Input: part model. Units: mm. Frame: model coordinates. A direction names the side the tool comes from. Coordinates: 2 decimals unless noted, no trailing zeros. Write each loop counter-clockwise with the first axis right and the second up, starting at its lowest first coordinate (ties: lowest second). Pieces come first, ordered by that corner, then holes.
1) Section query A-A (y = 12.5). Output: boundary loops of the cut face in (x, z).
2) Set-up query: faces 1 (the cylindrical face through (-1.08, -10.39, -4.88)), 2 (the cylindrical face through (-0.59, 12.89, 4.46)). Return all of +Z, -Z, +X, -X, +Y, -Y with unobstructed straight access to the full face (end or side cutting, diameter ignored); none if empty.
3) Section query B-B (y = -10.5). Output: boundary loops of the cut face in (x, z), then the cut area to 3 significant figures.
4) Line query: L1, parallel to Z at x = 0, y = -5; L2, parallel to Z at x = 0, y = 3.5; L3, parallel to X at y = -10, z = -0.75. Output: solid intervals per line, ascending.
5) Pin query (flat end, axial travel): pin 1 Ø5 at (x, y) = (-0.5, -12.5) entering from +Z; pin 2 Ø5 at (y, z) = (8.5, 2) entering from -X; pin 3 Ø3 at (x, z) = (-1.5, 4) entering from -Y; pin 4 Ø4 at (x, z) = (-1.5, 5.5) entering from +Y. Return the tip coordinate at first contact, or that it passes through.
from build123d import *

# Parameters (mm, degrees)
F0_R        = 7
F0_R_2      = 6.5
F0_R_3      = 6
F0_R_4      = 5.5
F0_R_5      = 5
F0_R_6      = 4.5
F0_R_7      = 4
F1_DEPTH    = 2
F2_DEPTH    = 4.5
F3_DEPTH    = 7
F4_DEPTH    = 9.5
F5_DEPTH    = 12
F6_DEPTH    = 14.5
F7_DEPTH    = 17
F8_R        = 3.25
F9_DEPTH    = 17
F10_SIZE2   = 0.692820323
F10_SIZE    = 0.4
F10_2_SIZE2 = 0.692820323
F10_2_SIZE  = 0.4
F10_3_SIZE2 = 0.692820323
F10_3_SIZE  = 0.4
F10_4_SIZE2 = 0.692820323
F10_4_SIZE  = 0.4
F10_5_SIZE2 = 0.692820323
F10_5_SIZE  = 0.4
F10_6_SIZE2 = 0.692820323
F10_6_SIZE  = 0.4


with BuildPart() as f1:
    # F0 (on Front) → F1 (new body)
    with BuildSketch(Plane.XZ):
        Circle(F0_R)
        Circle(F0_R_2, mode=Mode.SUBTRACT)
        Circle(F0_R_2)
        Circle(F0_R_3, mode=Mode.SUBTRACT)
        Circle(F0_R_3)
        Circle(F0_R_4, mode=Mode.SUBTRACT)
        Circle(F0_R_4)
        Circle(F0_R_5, mode=Mode.SUBTRACT)
        Circle(F0_R_5)
        Circle(F0_R_6, mode=Mode.SUBTRACT)
        Circle(F0_R_6)
        Circle(F0_R_7, mode=Mode.SUBTRACT)
        Circle(F0_R_7)
    extrude(amount=F1_DEPTH)

    # F0 (on Front) → F2 (join, through all)
    with BuildSketch(Plane.XZ):
        Circle(F0_R_2)
        Circle(F0_R_3, mode=Mode.SUBTRACT)
        Circle(F0_R_3)
        Circle(F0_R_4, mode=Mode.SUBTRACT)
        Circle(F0_R_4)
        Circle(F0_R_5, mode=Mode.SUBTRACT)
        Circle(F0_R_5)
        Circle(F0_R_6, mode=Mode.SUBTRACT)
        Circle(F0_R_6)
        Circle(F0_R_7, mode=Mode.SUBTRACT)
        Circle(F0_R_7)
    extrude(amount=F2_DEPTH)

    # F0 (on Front) → F3 (join, through all)
    with BuildSketch(Plane.XZ):
        Circle(F0_R_3)
        Circle(F0_R_4, mode=Mode.SUBTRACT)
        Circle(F0_R_4)
        Circle(F0_R_5, mode=Mode.SUBTRACT)
        Circle(F0_R_5)
        Circle(F0_R_6, mode=Mode.SUBTRACT)
        Circle(F0_R_6)
        Circle(F0_R_7, mode=Mode.SUBTRACT)
        Circle(F0_R_7)
    extrude(amount=F3_DEPTH)

    # F0 (on Front) → F4 (join, through all)
    with BuildSketch(Plane.XZ):
        Circle(F0_R_4)
        Circle(F0_R_5, mode=Mode.SUBTRACT)
        Circle(F0_R_5)
        Circle(F0_R_6, mode=Mode.SUBTRACT)
        Circle(F0_R_6)
        Circle(F0_R_7, mode=Mode.SUBTRACT)
        Circle(F0_R_7)
    extrude(amount=F4_DEPTH)

    # F0 (on Front) → F5 (join, through all)
    with BuildSketch(Plane.XZ):
        Circle(F0_R_5)
        Circle(F0_R_6, mode=Mode.SUBTRACT)
        Circle(F0_R_6)
        Circle(F0_R_7, mode=Mode.SUBTRACT)
        Circle(F0_R_7)
    extrude(amount=F5_DEPTH)

    # F0 (on Front) → F6 (join, through all)
    with BuildSketch(Plane.XZ):
        Circle(F0_R_6)
        Circle(F0_R_7, mode=Mode.SUBTRACT)
        Circle(F0_R_7)
    extrude(amount=F6_DEPTH)

    # F0 (on Front) → F7 (join, through all)
    with BuildSketch(Plane.XZ):
        Circle(F0_R_7)
    extrude(amount=F7_DEPTH)

    # F8 (on face) → F9 (cut, through all)
    with BuildSketch(Plane.XZ.offset(17)):
        Circle(F8_R)
    extrude(amount=-F9_DEPTH, mode=Mode.SUBTRACT)

    # F10
    f10_edges = [f1.edges().sort_by_distance(p)[0] for p in [
        (-5, -12, 0),
    ]]
    f10_side = f1.faces().sort_by_distance((-4.858579, -12, 0))[0]
    chamfer(f10_edges, length=F10_SIZE, length2=F10_SIZE2, reference=f10_side)

    # F10#2
    f10_2_edges = [f1.edges().sort_by_distance(p)[0] for p in [
        (-5.5, -9.5, 0),
    ]]
    f10_2_side = f1.faces().sort_by_distance((-5.344437, -9.5, 0))[0]
    chamfer(f10_2_edges, length=F10_2_SIZE, length2=F10_2_SIZE2, reference=f10_2_side)

    # F10#3
    f10_3_edges = [f1.edges().sort_by_distance(p)[0] for p in [
        (-6, -7, 0),
    ]]
    f10_3_side = f1.faces().sort_by_distance((-5.830294, -7, 0))[0]
    chamfer(f10_3_edges, length=F10_3_SIZE, length2=F10_3_SIZE2, reference=f10_3_side)

    # F10#4
    f10_4_edges = [f1.edges().sort_by_distance(p)[0] for p in [
        (-6.5, -4.5, 0),
    ]]
    f10_4_side = f1.faces().sort_by_distance((-6.316152, -4.5, 0))[0]
    chamfer(f10_4_edges, length=F10_4_SIZE, length2=F10_4_SIZE2, reference=f10_4_side)

    # F10#5
    f10_5_edges = [f1.edges().sort_by_distance(p)[0] for p in [
        (-4.5, -14.5, 0),
    ]]
    f10_5_side = f1.faces().sort_by_distance((-4.372721, -14.5, 0))[0]
    chamfer(f10_5_edges, length=F10_5_SIZE, length2=F10_5_SIZE2, reference=f10_5_side)

    # F10#6
    f10_6_edges = [f1.edges().sort_by_distance(p)[0] for p in [
        (-4, -17, 0),
    ]]
    f10_6_side = f1.faces().sort_by_distance((-3.886863, -17, 0))[0]
    chamfer(f10_6_edges, length=F10_6_SIZE, length2=F10_6_SIZE2, reference=f10_6_side)

    # F11: F1 across plane


with BuildPart() as f1_1:
    add(f1.part)
    add(f1.part.mirror(Plane.XZ))


solid = f1_1.part
Answer:
1. outline: circle Ø9 at (0, 0); hole circle Ø6.5 at (0, 0)
2. face 1: -Y
2. face 2: +Y
3. outline: circle Ø10 at (0, 0); hole circle Ø6.5 at (0, 0)
3. area: 45.4 mm2
4. L1: z = -6 to -3.25, 3.25 to 6
4. L2: z = -6.5 to -3.25, 3.25 to 6.5
4. L3: x = -4.94 to -3.16, 3.16 to 4.94
5. pin 1: stops at z = 5
5. pin 2: stops at x = -5.95
5. pin 3: stops at y = -17
5. pin 4: stops at y = 16.83
